Autodesk Inventor part; units mm, degrees
ref_plane "YZ Plane" through (0, 0, 0) normal (1, 0, 0) x (0, 1, 0)
ref_plane "XZ Plane" through (0, 0, 0) normal (0, 1, 0) x (-1, 0, 0)
ref_plane "XY Plane" through (0, 0, 0) normal (0, 0, 1) x (1, 0, 0)
sketch "Sketch1" plane through (0, 0, 0) normal (0, 0, 1) x (1, 0, 0)
  line L0 (0, -78.4) -> (0, 29.4)
  line L1 (5.5, 10.25) -> (5.5, 14)
  line L2 (5.5, 14) -> (10, 14)
  line L3 (10, 14) -> (10, -3)
  line L4 (10, -3) -> (2, -3)
  line L5 (2, -3) -> (2, -63)
  line L6 (2, -63) -> (0, -63)
  line L7 (-5.5, 10.25) -> (-5.5, 14)
  line L8 (-5.5, 14) -> (-10, 14)
  line L9 (-10, 14) -> (-10, -3)
  line L10 (-10, -3) -> (-2, -3)
  line L11 (-2, -3) -> (-2, -63)
  line L12 (-2, -63) -> (0, -63)
  arc A0 (-5.5, 10.25) -> (5.5, 10.25) centre (0, 10.25) ccw
  point P0 (0, 0)
  point P1 (5.5, 3.5)
  point P2 (-5.5, 3.5)
  point P3 (5.5, -3)
  point P4 (0, 14)
  dimension "d0" = 4.5
  dimension "d1" = 20
  dimension "d2" = 4
  dimension "d7" = 60
  dimension "d13" = 11
  dimension "d14" = 17
  dimension "d16" = 3.75
extrude "Extrusion1" add sketch "Sketch1" along normal blind 0.635
fillet "Fillet1" radius 1.25 4 edges at (-10, 14, 0.3175) (10, 14, 0.3175) (-5.5, 14, 0.3175) (5.5, 14, 0.3175)
fillet "Fillet3" radius 4 2 edges at (-10, -3, 0.3175) (10, -3, 0.3175)
fillet "Fillet4" radius 1.5 2 edges at (-2, -3, 0.3175) (2, -3, 0.3175)
properties part number "ASAP_Handle_Fixture_New2_1"
Input: part model. Units: mm. Frame: model coordinates. A direction names the side the tool comes from. Round coordinates to 2 decimals unless told otherwise and drop trailing zeros. Loops run counter-clockwise (first coordinate to the right, second up) from the corner with the lowest first, then second, coordinate; pieces in that order, holes last. Notation, with made-up numbers: (19, -30.5) - (74, -30.5) arc R13 cw to (74, -7.5) - close; hole circle Ø9 at (60, 88). An arc over 180 degrees is marked (long way). One line per item, written item: value. Start each with the question number.
(1) Draft query along X for faces 1 (the flat face through (0, -13, 0)), 2 (the cylindrical face through (0.12, 4.75, 0.31)), 3 (the cylindrical face through (-8.859, -1.797, 0.322)), 4 (the cylindrical face through (-5.856, 13.624, 0.322)). Return one class per face: +X half, -X half, draft (parallel to the pull), parting line (faces both ways), or undercut.
(2) Section A-A, the plane z = 0.35. Return loops of the section in (x, y), plus the area to 3 significant figures.
(3) Section B-B, the plane x = 0. Return loops of the section in (y, z) (3 decimals).
(4) Section C-C, the plane y = -51. Return loops of the section in (x, z) (3 decimals), plus the area to 3 significant figures.
(5) Access query for faces 5 (the cylindrical face through (5.876, 13.644, 0.322)), 6 (the cylindrical face through (-2.43, -3.45, 0.32)). Directions: +Z, -Z, +X, -X, +Y, -Y. A direction counts if a zero-diameter tool reaches every point of the face in a straight line with its end or side. Return the directions, or none.
(6) Ray query, line 1 (X direction, y = -6.5, z = 0.2); line 2 (Y direction, x = -3.5, z = 0.35); line 3 (X direction, y = 6.5, z = 0.5). Return the intervals inside material, ascending. Write a range as [from, to].
Results below:
1. face 1: draft
1. face 2: undercut
1. face 3: -X half
1. face 4: undercut
2. outline: (-10, 1) arc R4 ccw to (-6, -3) - (-3.5, -3) arc R1.5 cw to (-2, -4.5) - (-2, -63) - (2, -63) - (2, -4.5) arc R1.5 cw to (3.5, -3) - (6, -3) arc R4 ccw to (10, 1) - (10, 12.75) arc R1.25 ccw to (8.75, 14) - (6.75, 14) arc R1.25 ccw to (5.5, 12.75) - (5.5, 10.25) arc R5.5 cw to (-5.5, 10.25) - (-5.5, 12.75) arc R1.25 ccw to (-6.75, 14) - (-8.75, 14) arc R1.25 ccw to (-10, 12.75) - close
2. area: 484 mm^2
3. outline: (-63, 0) - (4.75, 0) - (4.75, 0.635) - (-63, 0.635) - close
4. outline: (-2, 0) - (2, 0) - (2, 0.635) - (-2, 0.635) - close
4. area: 2.54 mm^2
5. face 5: +Z, -Z, +Y
5. face 6: +Z, -Z, -X, -Y
6. line 1: [-2, 2]
6. line 2: [-3, 6.01]
6. line 3: [-10, -4.02], [4.02, 10]
